Can you work these out from the model? Positions are in its coordinate system, mm. A direction names the side the tool comes from. Coordinates: 2 decimals unless noted, no trailing zeros. Write each loop counter-clockwise with the first axis right and the second up, starting at its lowest first coordinate (ties: lowest second). Pieces come first, ordered by that corner, then holes. Notation, with made-up numbers: M -38.75,33 L 0.25,33 A34 ccw 0.25,72 Z; hole C 70,37 d11. An arc over 180 degrees is marked long. Answer as a JSON object with one key per item and string values. Group by question number.
from build123d import *

# Parameters (mm, degrees)
SKETCH1_R           = 17.5
BOSS_EXTRUDE1_DEPTH = 14
SKETCH2_R           = 4
CUT_EXTRUDE1_DEPTH  = 11


with BuildPart() as part:
    # Sketch1 → Boss-Extrude1 (new body)
    with BuildSketch(Plane.XY):
        with BuildLine():
            Line((40.87, -22.87), (-40.87, -22.87))
            Line((-40.87, -22.87), (-40.87, -12.87))
            Line((-40.87, -12.87), (-25.87, -12.87))
            ThreePointArc((-25.87, -12.87), (-23.748679656, -11.991320344), (-22.87, -9.87))
            Line((-22.87, -9.87), (-22.87, 0))
            ThreePointArc((-22.87, 0), (0, 22.87), (22.87, 0))
            Line((22.87, 0), (22.87, -9.87))
            ThreePointArc((22.87, -9.87), (23.748679656, -11.991320344), (25.87, -12.87))
            Line((25.87, -12.87), (40.87, -12.87))
            Line((40.87, -12.87), (40.87, -22.87))
        make_face()
        Circle(SKETCH1_R, mode=Mode.SUBTRACT)
    extrude(amount=BOSS_EXTRUDE1_DEPTH)

    # Sketch2 → Cut-Extrude1 (cut, through all)
    with BuildSketch(Plane(origin=(0, -12.87, 0), x_dir=(1, 0, 0), z_dir=(0, 1, 0))):
        with Locations((33.37, -7.5)):
            Circle(SKETCH2_R)
    cut_extrude1 = extrude(amount=-CUT_EXTRUDE1_DEPTH, mode=Mode.SUBTRACT)

    # Mirror1: Cut-Extrude1 across plane
    add(cut_extrude1.mirror(Plane(origin=(0, 0, 0), x_dir=(0, 0, 1), z_dir=(1, 0, 0))), mode=Mode.SUBTRACT)


solid = part.part
Q1. Please list where these lines run through material, in increasing order: L1, parallel to Y at x = 0, z = 11; L2, parallel to Z at x = -33.37, y = -19.75; L3, parallel to X at y = -19.5, z = 7.5.
Q2. If we section it at B-B on z = 7.5: List the corners of the cut face in (x, y) for me.
Q3. If we section it at A-A on x = 33.37: List the corners of the cut face in (y, z) for me, and give its area (3 significant figures).
Q4. If we section it at D-D on y = 5: List the corners of the cut face in (x, z) for me.
Q5. If we section it at C-C on y = -16: List the corners of the cut face in (x, z) for me.
Q6. On a 3-axis mill with a long thin cutter (end or side, diameter ignored), from which of +Z, -Z, +X, -X, +Y, -Y can I reach the whole of each face in a straight line? I mean faces 5 (the cylindrical face through (-29.374, -17.8, 7.324)), 6 (the flat face through (30, -12.87, 5)), 7 (the flat face through (-22.87, -5, 7)). Say none if no direction works.
Q7. We'd pull the mould along Y, two halves only. Please class faces 1 (the cylindrical face through (-13.887, -10.648, 6.902)), 2 (the flat face through (1, -22.87, 7)), 3 (the flat face through (-37, -12.87, 5)), 4 (the flat face through (10, -15, 0)): pulls with the +Y half, pulls with the -Y half, needs draft (parallel to the pull), parting line crosses it, or undercut.
Q8. Will these pins go through, and if not, where does the flat tip stop? pin 1 (4 mm diameter, centred on x = -33.5, z = 4.5, fed in from +Y); pin 2 (2 mm diameter, centred on x = -4.5, y = 17, fed in from -Z); pin 3 (1.5 mm diameter, centred on x = 19.5, z = 5, fed in from +Y); pin 4 (6 mm diameter, centred on y = -6.5, z = 12.5, fed in from -X).
Reply:
{
 "1": {"L1": "-22.87 to -17.5, 17.5 to 22.87", "L2": "0 to 3.5, 11.5 to 14", "L3": "-40.87 to -37.37, -29.37 to 29.37, 37.37 to 40.87"},
 "2": {"outline": "M -40.87,-22.87 L -37.37,-22.87 L -37.37,-12.87 L -40.87,-12.87 Z; M -29.37,-22.87 L 29.37,-22.87 L 29.37,-12.87 L 25.87,-12.87 A3 cw 22.87,-9.87 L 22.87,0 A22.87 ccw -22.87,0 L -22.87,-9.87 A3 cw -25.87,-12.87 L -29.37,-12.87 Z; M 37.37,-22.87 L 40.87,-22.87 L 40.87,-12.87 L 37.37,-12.87 Z; hole C 0,0 d35"},
 "3": {"outline": "M -22.87,0 L -12.87,0 L -12.87,3.5 L -22.87,3.5 Z; M -22.87,11.5 L -12.87,11.5 L -12.87,14 L -22.87,14 Z", "area": "60.0 mm^2"},
 "4": {"outline": "M -22.32,0 L -16.77,0 L -16.77,14 L -22.32,14 Z; M 16.77,0 L 22.32,0 L 22.32,14 L 16.77,14 Z"},
 "5": {"outline": "M -40.87,0 L -7.09,0 L -7.09,14 L -40.87,14 Z; M 7.09,0 L 40.87,0 L 40.87,14 L 7.09,14 Z; hole C -33.37,7.5 d8; hole C 33.37,7.5 d8"},
 "6": {"face 5": "+Y, -Y", "face 6": "+Z, -Z, +X, +Y", "face 7": "+Z, -Z, -X, +Y"},
 "7": {"face 1": "undercut", "face 2": "pulls with the -Y half", "face 3": "pulls with the +Y half", "face 4": "needs draft"},
 "8": {"pin 1": "y = -12.87", "pin 2": "z = 0", "pin 3": "y = 13.09", "pin 4": "x = -22.87"}
}
